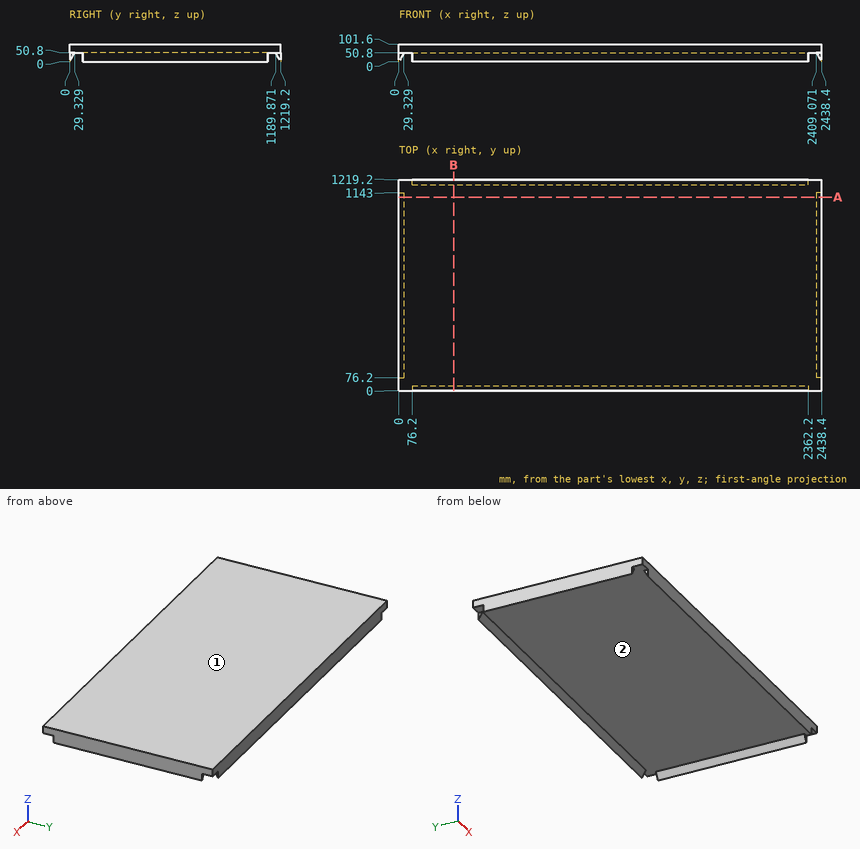
Verification items for this drawing (mm, ordinates from the low corner). A direction names the side the tool comes from. Give positions to 0.01 mm unless a question says otherwise; leave off trailing zeros. Loops run counter-clockwise (first coordinate to the right, second up) from the corner with the lowest first, then second, coordinate; pieces in that order, holes last. Notation, with made-up numbers: M -9.5,-34 L 19.5,-34 A15 ccw 19.5,-29 Z; hole C -5.75,-19 d9. An arc over 180 degrees is marked long. Return JSON: item names as keys, results as strings. Group by question number.
1. Go/stop test with flat-tipped pins: pin 1 (14.5 mm diameter, centred on x = 2421, z = 30, fed in from -Y); pin 2 (14.5 mm diameter, centred on y = 1206, z = 32.5, fed in from +X); pin 3 (23.5 mm diameter, centred on x = 18, z = 36, fed in from +Y). Record where each tip stops, or that it passes through.
2. Cross-section at A-A on y = 1118. Record the boundary of the cut face in (x, z).
3. Tool access check on the marked faces 1 and 2. Record the directions out of +Z, -Z, +X, -X, +Y, -Y that give a thin tool (end or side, any length) a straight path to the whole face; none if there is none.
4. Cross-section at B-B on x = 316.5. Record the boundary of the cut face in (y, z), plus the area to 3 significant figures.
5. Thickness scan on L1, parallel to X at y = 635.5, z = 47 (1 decimal); L2, parallel to Z at x = 1803, y = 94.5; L3, parallel to Y at x = 2183.5, z = 19.5. Record the ranges inside material, lowest first.
Return value:
{
 "1": {"pin 1": "y = 76.2", "pin 2": "x = 2362.2", "pin 3": "y = 1143"},
 "2": {"outline": "M 0,0 L 29.33,50.8 L 2409.07,50.8 L 2438.4,0 L 2438.4,101.6 L 0,101.6 Z"},
 "3": {"face 1": "+Z, +X, -X, +Y, -Y", "face 2": "-Z"},
 "4": {"outline": "M 0,0 L 29.33,50.8 L 1189.87,50.8 L 1219.2,0 L 1219.2,101.6 L 0,101.6 Z", "area": "63,400 mm^2"},
 "5": {"L1": "0 to 27.1, 2411.3 to 2438.4", "L2": "50.8 to 101.6", "L3": "0 to 11.26, 1207.94 to 1219.2"}
}
